Model file for the job. Use its own axes, mm. Face numbers are marked on the shaded views. Coordinates: 2 decimals unless noted, no trailing zeros. Order: outer loops, then holes, each group sorted by start corner. A loop starts at its lowest first (then second) coordinate and runs counter-clockwise, first axis right, second up. Notation, with made-up numbers: (35, -29) -> (54, -29) arc R28 cw to (54, -1) -> close; hole circle Ø3 at (-11.5, -37.5). An arc over 180 degrees is marked (long way). Return JSON: item names as keys, results as strings. Group by question number.
1) Cut at D-D (x = -87). Write the cut outline in (y, z).
2) Cut at B-B (z = 7.5). Write the cut outline in (x, y) (3 decimals), and give its area (3 significant figures).
3) Probe line 1 (Y direction, x = -90, z = 7.75); line 2 (X direction, y = -1.5, z = 9.75); line 3 (X direction, y = 0.25, z = 16.75). List the from-to ranges inside material, lowest first.
4) Cut at A-A (x = -90). Write the cut outline in (y, z), and give its area (3 significant figures).
5) Flat gauge pins, fed straight in: pin 1 (1 mm diameter, centred on y = 2, z = 20.5, fed in from -X); pin 2 (3.5 mm diameter, centred on x = -90, y = 0, fed in from +Z). Where does each tip first touch, or does it go through?
6) Pull direction Y, two halves, no side cores. Call the marked faces 1, 2 and 3: +Y half, -Y half, draft (parallel to the pull), parting line (faces both ways), or undercut.
7) Cut at C-C (y = 0.5). Write the cut outline in (x, z), and give its area (3 significant figures).
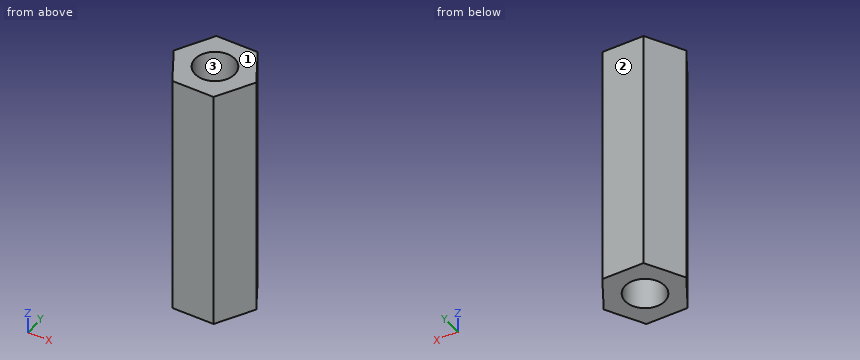
from build123d import *

# Parameters (mm, degrees)
CYLINDER013_R     = 2
CYLINDER013_DEPTH = 50
PAD_DEPTH         = 25


with BuildPart() as cylinder013:
    # Cylinder013 → Cylinder013 (new body)
    with BuildSketch(Plane(origin=(-90, 0, -10), x_dir=(1, 0, 0), z_dir=(0, 0, 1))):
        Circle(CYLINDER013_R)
    extrude(amount=CYLINDER013_DEPTH)


with BuildPart() as obj1:
    # Polygon → Pad (new body)
    with BuildSketch(Plane(origin=(-90, 0, 0), x_dir=(1, 0, 0), z_dir=(0, 0, 1))):
        Polygon((2.075, 3.594005), (4.15, 0), (2.075, -3.594005), (-2.075, -3.594005), (-4.15, 0), (-2.075, 3.594005), align=None)
    extrude(amount=PAD_DEPTH)

    # Cut002002: cut Cylinder013
    add(cylinder013.part, mode=Mode.SUBTRACT)


solid = obj1.part
Answers below:
{
 "1": {"outline": "(-1.99, 0) -> (1.99, 0) -> (1.99, 25) -> (-1.99, 25) -> close"},
 "2": {"outline": "(-94.15, 0) -> (-92.075, -3.594) -> (-87.925, -3.594) -> (-85.85, 0) -> (-87.925, 3.594) -> (-92.075, 3.594) -> close; hole circle Ø4 at (-90, 0)", "area": "32.2 mm^2"},
 "3": {"line 1": "y = -3.59 to -2, 2 to 3.59", "line 2": "x = -93.28 to -91.32, -88.68 to -86.72", "line 3": "x = -94.01 to -91.98, -88.02 to -85.99"},
 "4": {"outline": "(-3.59, 0) -> (-2, 0) -> (-2, 25) -> (-3.59, 25) -> close; (2, 0) -> (3.59, 0) -> (3.59, 25) -> (2, 25) -> close", "area": "79.7 mm^2"},
 "5": {"pin 1": "stops at x = -93.28", "pin 2": "passes through"},
 "6": {"face 1": "draft", "face 2": "+Y half", "face 3": "undercut"},
 "7": {"outline": "(-93.86, 0) -> (-91.94, 0) -> (-91.94, 25) -> (-93.86, 25) -> close; (-88.06, 0) -> (-86.14, 0) -> (-86.14, 25) -> (-88.06, 25) -> close", "area": "96.2 mm^2"}
}
